Verification items for the finished model (mm, model axes). A direction names the side the tool comes from. Coordinates: 2 decimals unless noted, no trailing zeros. Order: outer loops, then holes, each group sorted by start corner. A loop starts at its lowest first (then second) coordinate and runs counter-clockwise, first axis right, second up. Notation, with made-up numbers: (66.5, -29.75) -> (74.5, -29.75) arc R19 ccw to (74.5, -2.75) -> close; hole circle Ø9 at (55.5, 71). An arc over 180 degrees is marked (long way). Write each question's results on one line, items separated by ' | '. Start each with the question number.
(1) Cross-section at D-D on x = 9. Enter the section's corners in (y, z), and give its area (3 significant figures).
(2) Cross-section at B-B on x = 18.5. Enter the section's corners in (y, z), and give its area (3 significant figures).
(3) Draft check along X on faces 1 (the cylindrical face through (18.044, 0.493, 9.905)), 2 (the flat face through (20, 3, 6)), 3 (the flat face through (12, 5.5, 3)). Enter one of: +X half, -X half, draft (parallel to the pull), parting line (faces both ways), or undercut.
(4) Go/stop test with flat-tipped pins: pin 1 (1.8 mm diameter, centred on x = 1.5, z = 10.5, fed in from +Y); pin 2 (1 mm diameter, centred on x = 1.5, z = 1.5, fed in from +Y). Record where each tip stops, or that it passes through.
(5) Thickness scan on probe 1 along X at (y, z) = (1.75, 6); probe 2 along X at (y, z) = (4.3, 1.5); probe 3 along Z at (x, y) = (15.5, 2.4). Record the ranges inside material, lowest first. Write a range as [from, to].
(6) Cross-section at A-A on z = 1.5. Enter the section's corners in (x, y).
(7) Cross-section at C-C on y = 1.95. Give the number of separate pieces and of enclosed holes in the cut face, and give its area (3 significant figures).
(8) Set-up check for faces 4 (the flat face through (0, 3, 6)), 5 (the cylindrical face through (17.648, 0.789, 6.107)), 6 (the cylindrical face through (17.524, 3.282, 10.283)): record each of +Z, -Z, +X, -X, +Y, -Y from which the full face is reachable in a straight line by a thin tool's end or side.
```python
from build123d import *

# Parameters (mm, degrees)
SKETCH_1_W               = 20
SKETCH_1_H               = 12
SKETCH_1_R               = 3.5
EXTRUDE_1_DEPTH          = 5.5
SKETCH_1_17_R            = 2.65
CUT_EXTRUDE_8_DEPTH      = 1.6
CUT_EXTRUDE_3_DEPTH      = 24.963513933
CUT_EXTRUDE_3_DEPTH_BACK = 24.963513933
SKETCH_3_R               = 0.75
SKETCH_3_R_2             = 0.35
CUT_EXTRUDE_START        = 5.5
SKETCH_3_5_R             = 1
CUT_EXTRUDE_4_DEPTH      = 4.5


with BuildPart() as part:
    # 草图1 → 凸台-拉伸1 (new body)
    with BuildSketch(Plane(origin=(0, 0, 0), x_dir=(1, 0, 0), z_dir=(0, 1, 0))):
        with Locations((10, -6)):
            Rectangle(SKETCH_1_W, SKETCH_1_H)
        with Locations(Location((9, -6, 0), (0, 0, 270))):
            Circle(SKETCH_1_R, mode=Mode.SUBTRACT)
    extrude(amount=EXTRUDE_1_DEPTH)

    # 草图1<17> → 切除-拉伸8 (cut)
    with BuildSketch(Plane(origin=(0, 0, 0), x_dir=(1, 0, 0), z_dir=(0, 1, 0))):
        with Locations((15, -6)):
            Circle(SKETCH_1_17_R)
    extrude(amount=CUT_EXTRUDE_8_DEPTH, mode=Mode.SUBTRACT)

    # 草图3 → 切除-拉伸3 (cut, two sides: drawn at the far end of the back side and taken through both)
    with BuildSketch(Plane(origin=(0, 0, 0), x_dir=(1, 0, 0), z_dir=(0, 1, 0)).offset(-CUT_EXTRUDE_3_DEPTH_BACK)):
        with Locations(Location((1.5, -1.5, 0), (0, 0, 270))):
            Circle(SKETCH_3_R)
        with Locations(Location((18.5, -1.5, 0), (0, 0, 270))):
            Circle(SKETCH_3_R)
        with Locations(Location((1.5, -10.5, 0), (0, 0, 270))):
            Circle(SKETCH_3_R)
        with Locations(Location((18.5, -10.5, 0), (0, 0, 270))):
            Circle(SKETCH_3_R)
        with Locations(Location((15.5, -3, 0), (0, 0, 270))):
            Circle(SKETCH_3_R_2)
        with Locations(Location((2.5, -6, 0), (0, 0, 270))):
            Circle(SKETCH_3_R_2)
        with Locations(Location((15.5, -9, 0), (0, 0, 270))):
            Circle(SKETCH_3_R_2)
    extrude(amount=CUT_EXTRUDE_3_DEPTH + CUT_EXTRUDE_3_DEPTH_BACK, mode=Mode.SUBTRACT)

    # 草图3<5> → 切除-拉伸4 (cut)
    with BuildSketch(Plane(origin=(0, 0, 0), x_dir=(1, 0, 0), z_dir=(0, 1, 0)).offset(CUT_EXTRUDE_START)):
        with Locations(Location((1.5, -1.5, 0), (0, 0, 270))):
            Circle(SKETCH_3_5_R)
        with Locations(Location((18.5, -1.5, 0), (0, 0, 270))):
            Circle(SKETCH_3_5_R)
        with Locations(Location((18.5, -10.5, 0), (0, 0, 270))):
            Circle(SKETCH_3_5_R)
        with Locations(Location((1.5, -10.5, 0), (0, 0, 270))):
            Circle(SKETCH_3_5_R)
    extrude(amount=-CUT_EXTRUDE_4_DEPTH, mode=Mode.SUBTRACT)


solid = part.part
```
Results are:
1) outline: (0, 0) -> (5.5, 0) -> (5.5, 2.5) -> (0, 2.5) -> close; (0, 9.5) -> (5.5, 9.5) -> (5.5, 12) -> (0, 12) -> close | area: 27.5 mm2
2) outline: (0, 0) -> (5.5, 0) -> (5.5, 0.5) -> (1, 0.5) -> (1, 0.75) -> (0, 0.75) -> close; (0, 2.25) -> (1, 2.25) -> (1, 2.5) -> (5.5, 2.5) -> (5.5, 9.5) -> (1, 9.5) -> (1, 9.75) -> (0, 9.75) -> close; (0, 11.25) -> (1, 11.25) -> (1, 11.5) -> (5.5, 11.5) -> (5.5, 12) -> (0, 12) -> close | area: 45.0 mm2
3) face 1: undercut | face 2: +X half | face 3: draft
4) pin 1: stops at y = 1 | pin 2: passes through
5) probe 1: x = [0, 2.15], [2.85, 5.5], [12.5, 20] | probe 2: x = [0, 0.5], [2.5, 17.5], [19.5, 20] | probe 3: z = [0, 2.65], [3.35, 8.65], [9.35, 12]
6) outline: (0, 0) -> (0.75, 0) -> (0.75, 1) -> (0.5, 1) -> (0.5, 5.5) -> (0, 5.5) -> close; (2.25, 0) -> (17.75, 0) -> (17.75, 1) -> (17.5, 1) -> (17.5, 5.5) -> (2.5, 5.5) -> (2.5, 1) -> (2.25, 1) -> close; (19.25, 0) -> (20, 0) -> (20, 5.5) -> (19.5, 5.5) -> (19.5, 1) -> (19.25, 1) -> close
7) separate pieces: 1 | enclosed holes: 8 | area: 188 mm2
8) face 4: +Z, -Z, -X, +Y, -Y | face 5: -Y | face 6: +Y
